Design review of the part built by this model. Coordinates are the model's own, in mm. Give positions to 0.01 mm unless a question says otherwise; leave off trailing zeros. Loops run counter-clockwise (first coordinate to the right, second up) from the corner with the lowest first, then second, coordinate; pieces in that order, holes last.
from build123d import *

# Parameters (mm, degrees)
SKETCH1_R           = 1.85
SKETCH1_R_2         = 4
BOSS_EXTRUDE1_DEPTH = 2


with BuildPart() as part:
    # Sketch1 → Boss-Extrude1 (new body)
    with BuildSketch(Plane(origin=(0, 2, 0), x_dir=(1, 0, 0), z_dir=(0, 1, 0))):
        with BuildLine():
            Line((64, 13.5), (0, 13.5))
            ThreePointArc((0, 13.5), (-13.5, 0), (0, -13.5))
            Line((0, -13.5), (64, -13.5))
            ThreePointArc((64, -13.5), (77.5, 0), (64, 13.5))
        make_face()
        with Locations((56, 0)):
            Circle(SKETCH1_R, mode=Mode.SUBTRACT)
        with Locations((64, -8)):
            Circle(SKETCH1_R, mode=Mode.SUBTRACT)
        with Locations((72, 0)):
            Circle(SKETCH1_R, mode=Mode.SUBTRACT)
        with Locations((64, 8)):
            Circle(SKETCH1_R, mode=Mode.SUBTRACT)
        with Locations((64, 0)):
            Circle(SKETCH1_R_2, mode=Mode.SUBTRACT)
        with Locations((-8, 0)):
            Circle(SKETCH1_R, mode=Mode.SUBTRACT)
        with Locations((0, -8)):
            Circle(SKETCH1_R, mode=Mode.SUBTRACT)
        with Locations((8, 0)):
            Circle(SKETCH1_R, mode=Mode.SUBTRACT)
        with Locations((0, 8)):
            Circle(SKETCH1_R, mode=Mode.SUBTRACT)
        Circle(SKETCH1_R_2, mode=Mode.SUBTRACT)
    extrude(amount=-BOSS_EXTRUDE1_DEPTH)


solid = part.part
Q1. Insertion check: pin 1 (3 mm diameter, centred on x = 41, z = 0, fed in from -Y). The pin has a flat end and moves straight along its axis. Give the tip position at first contact, or say it passes through.
Results:
pin 1: stops at y = 0
Q2. Draft analysis for pull direction X (two halves, no side actions). For faces 1 (the face through (32, 1, -13.5)), 2 (the face through (-13.497, 1.014, -0.297)), 3 (the face through (67.695, 1.014, 1.532)), state which applies: pulls with the +X half, pulls with the -X half, needs draft (parallel to the pull), parting line crosses it, or undercut.
Results:
face 1: needs draft
face 2: pulls with the -X half
face 3: undercut
Q3. Take a section at D-D (x = 72). Give the boundary of the cut face in (y, z), plus the area to 3 significant figures.
Results:
outline: (0, -10.87) - (2, -10.87) - (2, -1.85) - (0, -1.85) - close; (0, 1.85) - (2, 1.85) - (2, 10.87) - (0, 10.87) - close
area: 36.1 mm2
Q4. Take a section at C-C (z = -8). Give the boundary of the cut face in (x, y).
Results:
outline: (-10.87, 0) - (-1.85, 0) - (-1.85, 2) - (-10.87, 2) - close; (1.85, 0) - (62.15, 0) - (62.15, 2) - (1.85, 2) - close; (65.85, 0) - (74.87, 0) - (74.87, 2) - (65.85, 2) - close
Q5. Wall thickness on line 1 (Z direction, x = 64, y = 1.4); line 2 (X direction, y = 1, z = 8); line 3 (X direction, y = 0.7, z = 7.25): over which ranges is each line inside the solid? List them lowest first.
Results:
line 1: z = -13.5 to -9.85, -6.15 to -4, 4 to 6.15, 9.85 to 13.5
line 2: x = -10.87 to -1.85, 1.85 to 62.15, 65.85 to 74.87
line 3: x = -11.39 to -1.69, 1.69 to 62.31, 65.69 to 75.39
Q6. Take a section at A-A (z = 0). Give the boundary of the cut face in (x, y), plus the area to 3 significant figures.
Results:
outline: (-13.5, 0) - (-9.85, 0) - (-9.85, 2) - (-13.5, 2) - close; (-6.15, 0) - (-4, 0) - (-4, 2) - (-6.15, 2) - close; (4, 0) - (6.15, 0) - (6.15, 2) - (4, 2) - close; (9.85, 0) - (54.15, 0) - (54.15, 2) - (9.85, 2) - close; (57.85, 0) - (60, 0) - (60, 2) - (57.85, 2) - close; (68, 0) - (70.15, 0) - (70.15, 2) - (68, 2) - close; (73.85, 0) - (77.5, 0) - (77.5, 2) - (73.85, 2) - close
area: 120 mm2
Q7. Take a section at B-B (x = 8). Give the boundary of the cut face in (y, z).
Results:
outline: (0, -13.5) - (2, -13.5) - (2, -1.85) - (0, -1.85) - close; (0, 1.85) - (2, 1.85) - (2, 13.5) - (0, 13.5) - close
